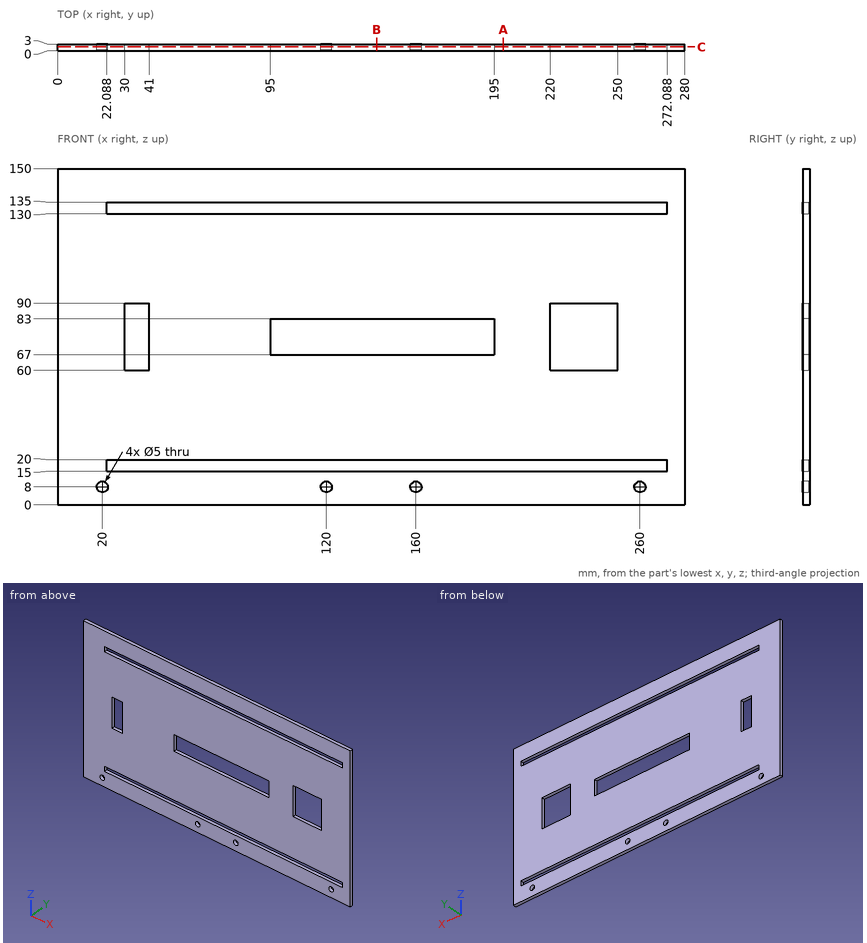
Job drawing, mm, ordinate dimensions from the low corner. One solid piece. Coordinates: 2 decimals unless noted, no trailing zeros. Loops run counter-clockwise (first coordinate to the right, second up) from the corner with the lowest first, then second, coordinate; pieces in that order, holes last. Notation, with made-up numbers: (-33, 60.5) - (-1, 60.5) arc R23 ccw to (-1, 83.5) - close; hole circle Ø2 at (62, -3). An arc over 180 degrees is marked (long way). Write item = value, one per line. Start each with the question number.
Q1. Cut at A-A, the plane x = 199. List the corners of the cut face in (y, z).
Q2. Cut at C-C, the plane y = 1.7. Give the number of separate pieces and of enclosed holes in the cut face, then the cut area to 3 significant figures.
Q3. Drill centre lines: L1, parallel to X at y = 1.2, z = 76.5; L2, parallel to Z at x = 96, y = 0.2; L3, parallel to X at y = 0.65, z = 8. Where is each one in solid material? Low to high.
Q4. Cut at B-B, the plane x = 142.5. List the corners of the cut face in (y, z).
Q5. Flat gauge pin, fed straight in: pin 1 Ø3 at (x, z) = (260, 8) entering from -Y. Where does the tip first touch, or does it go through?
Computed:
q1.outline = (0, 0) - (3, 0) - (3, 15) - (0, 15) - close; (0, 20) - (3, 20) - (3, 130) - (0, 130) - close; (0, 135) - (3, 135) - (3, 150) - (0, 150) - close
q2.separate_pieces = 1
q2.enclosed_holes = 9
q2.area = 36,600 mm²
q3.L1 = 0 to 30, 41 to 95, 195 to 220, 250 to 280
q3.L2 = 0 to 15, 20 to 67, 83 to 130, 135 to 150
q3.L3 = 0 to 17.5, 22.5 to 117.5, 122.5 to 157.5, 162.5 to 257.5, 262.5 to 280
q4.outline = (0, 0) - (3, 0) - (3, 15) - (0, 15) - close; (0, 20) - (3, 20) - (3, 67) - (0, 67) - close; (0, 83) - (3, 83) - (3, 130) - (0, 130) - close; (0, 135) - (3, 135) - (3, 150) - (0, 150) - close
q5.pin_1 = through
